CAD build for the part. Positions are in the model's coordinates, mm. A direction names the side the tool comes from. Coordinates: 2 decimals unless noted, no trailing zeros. Order: outer loops, then holes, each group sorted by start corner. A loop starts at its lowest first (then second) coordinate and runs counter-clockwise, first axis right, second up. Notation, with made-up numbers: (29.5, 43.5) - (75.5, 43.5) arc R4 cw to (75.5, 49.5) - close; hole circle Ø3 at (-5.75, -38.75). An arc over 180 degrees is marked (long way). Return JSON: item names as keys, results as strings.
from build123d import *

# Parameters (mm, degrees)
CUT_EXTRUDE1_START     = -100
CUT_EXTRUDE1_DEPTH     = 100
F_1_12_TAPPED_HOLE1_D  = 23.41626
F_1_1_DIAMETER_HOLE1_D = 25.4
CHAMFER1_SIZE          = 1


with BuildPart() as part:
    # Sketch2 one side → Revolve1 (revolve)
    with BuildSketch(Plane.XY, mode=Mode.PRIVATE) as revolve1_sk:
        with BuildLine():
            Line((-94, 50), (-94, 48.5))
            Line((-94, 48.5), (-97, 48.5))
            Line((-97, 48.5), (-97, 50))
            Line((-97, 50), (-100, 50))
            Line((-100, 50), (-100, 0))
            Line((-100, 0), (100, 0))
            Line((100, 0), (100, 50))
            Line((100, 50), (-16.67, 50))
            ThreePointArc((-16.67, 50), (-23.741067812, 52.928932188), (-26.67, 60))
            Line((-26.67, 60), (-26.67, 75))
            Line((-26.67, 75), (-60, 75))
            Line((-60, 75), (-60, 50))
            Line((-60, 50), (-94, 50))
        make_face()
    revolve(revolve1_sk.sketch.rotate(Axis((-100, 0, 0), (1, 0, 0)), 90), axis=Axis((-100, 0, 0), (1, 0, 0)))

    # Sketch3 → Cut-Extrude1 (cut)
    with BuildSketch(Plane(origin=(100, 0, 0), x_dir=(0, 0, -1), z_dir=(1, 0, 0)).offset(CUT_EXTRUDE1_START)):
        with BuildLine():
            ThreePointArc((33.071891388, 37.5), (0, 50), (-33.071891388, 37.5))
            Line((-33.071891388, 37.5), (33.071891388, 37.5))
        make_face()
        with BuildLine():
            Line((33.071891388, -37.5), (-33.071891388, -37.5))
            ThreePointArc((-33.071891388, -37.5), (0, -50), (33.071891388, -37.5))
        make_face()
    extrude(amount=CUT_EXTRUDE1_DEPTH, mode=Mode.SUBTRACT)

    # 1-12 Tapped Hole1 (through all)
    with Locations(Plane(origin=(0, 37.5, 0), x_dir=(1, 0, 0), z_dir=(0, 1, 0))):
        with Locations((50, 0)):
            Hole(F_1_12_TAPPED_HOLE1_D / 2)

    # 1 (1) Diameter Hole1 (through all)
    with Locations(Plane(origin=(100, 0, 0), x_dir=(0, 0, -1), z_dir=(1, 0, 0))):
        with Locations((0, 0)):
            Hole(F_1_1_DIAMETER_HOLE1_D / 2)

    # Chamfer1
    chamfer1_edges = [part.edges().sort_by_distance(p)[0] for p in [
        (-97, 0, -48.5),
        (100, 0, -50),
        (100, 20.571891388, 45.571891388),
    ]]
    chamfer(chamfer1_edges, length=CHAMFER1_SIZE)


solid = part.part
Item 1: Band-saw the part on C-C, the plane x = 16. List the corners of the cut face in (y, z).
Findings below:
{"outline": "(-37.5, -33.07) arc R50 ccw to (37.5, -33.07) - (37.5, 33.07) arc R50 ccw to (-37.5, 33.07) - close; hole circle Ø25.4 at (0, 0)"}
Item 2: Which spindle directions (+Z, -Z, +X, -X, +Y, -Y) get a long thin tool onto all of the face, cutting with end or side? Do faces 4 (the flat face through (0, 42, 0)), 5 (the flat face through (38, -37.5, 0)), 6 (the flat face through (-97, -11.3, 48.4)), 7 (the cylindrical face through (-98.52, -15.02, 47.69)). Say none if no direction does.
Findings below:
{"face 4": "+Z, -Z, +X, +Y", "face 5": "+Z, -Z, +X, -Y", "face 6": "none", "face 7": "-X"}
Item 3: Mould opens along Z. For faces 1 (the flat face through (38, 37.5, 0)), 2 (the conical face through (99.84, -0.6, -49.156)), 3 (the cylindrical face through (58.63, 24.6, -7.91)) say: released by +Z, released by -Z, zero draft, split by the parting line, or undercut.
Findings below:
{"face 1": "zero draft", "face 2": "released by -Z", "face 3": "undercut"}
Item 4: Band-saw the part on A-A, the plane x = 50. List the corners of the cut face in (y, z), then the cut area to 3 significant figures.
Findings below:
{"outline": "(-37.5, -33.07) arc R50 ccw to (37.5, -33.07) - (37.5, -11.71) - (4.92, -11.71) arc R12.7 cw to (-4.92, -11.71) - (-37.5, -11.71) - close; (-37.5, 11.71) - (-4.92, 11.71) arc R12.7 cw to (4.92, 11.71) - (37.5, 11.71) - (37.5, 33.07) arc R50 ccw to (-37.5, 33.07) - close", "area": "4,950 mm²"}
Item 5: Wall check: L1, parallel to Y at x = 8, z = 0; L2, parallel to X at y = 36.5, z = -60; L3, parallel to Y at x = -49.5, z = -10. Give the ranges that are in metal, low to high. Write a range as [from, to].
Findings below:
{"L1": "y = [-37.5, -12.7], [12.7, 37.5]", "L2": "x = [-60, -26.67]", "L3": "y = [-74.33, -7.83], [7.83, 74.33]"}
Item 6: Drop flat-ended pins along their axis: P1, Ø1.5, axis at x = -46.5, z = -18, coming from the -Y side; P2, Ø20, axis at x = 58, z = 15, coming from the +Y side; P3, Ø10, axis at x = 53, y = -13, coming from the +Z side. Give the stop position or say it passes through.
Findings below:
{"P1": "stops at y = -72.99", "P2": "stops at y = 37.5", "P3": "stops at z = 49.36"}
Item 7: Band-saw the part on D-D, the plane z = 0. Count the separate pieces of the cut face and the enclosed holes in it, then the cut area to 3 significant figures.
Findings below:
{"separate pieces": "4", "enclosed holes": "0", "area": "13,000 mm²"}
